from build123d import *

# Parameters (mm, degrees)
SKETCH1_W           = 45
SKETCH1_H           = 70
BOSS_EXTRUDE1_DEPTH = 3
SKETCH2_R           = 10.95
SKETCH2_W           = 24
SKETCH2_H           = 35
CUT_EXTRUDE1_DEPTH  = 4
SKETCH4_W           = 10
SKETCH4_H           = 3
BOSS_EXTRUDE3_DEPTH = 3
SKETCH3_W           = 3
SKETCH3_H           = 14
BOSS_EXTRUDE2_DEPTH = 3
SKETCH5_W           = 45
SKETCH5_H           = 55
BOSS_EXTRUDE4_DEPTH = 3
FILLET1_R           = 4
SKETCH6_R           = 15.5
CUT_EXTRUDE2_DEPTH  = 10


with BuildPart() as part:
    # Sketch1 → Boss-Extrude1 (new body)
    with BuildSketch(Plane.XY):
        Rectangle(SKETCH1_W, SKETCH1_H)
    extrude(amount=BOSS_EXTRUDE1_DEPTH)

    # Sketch2 → Cut-Extrude1 (cut, through all)
    with BuildSketch(Plane.XY.offset(3)):
        with Locations((0, 16)):
            Circle(SKETCH2_R)
        with Locations((0, -17.5)):
            Rectangle(SKETCH2_W, SKETCH2_H)
    extrude(amount=-CUT_EXTRUDE1_DEPTH, mode=Mode.SUBTRACT)

    # Sketch4 → Boss-Extrude3 (add)
    with BuildSketch(Plane.XY.offset(3)):
        with Locations((-10, 36.5)):
            Rectangle(SKETCH4_W, SKETCH4_H)
        with Locations((10, 36.5)):
            Rectangle(SKETCH4_W, SKETCH4_H)
    extrude(amount=-BOSS_EXTRUDE3_DEPTH)

    # Sketch3 → Boss-Extrude2 (add)
    with BuildSketch(Plane(origin=(0, 0, 0), x_dir=(-1, 0, 0), z_dir=(0, 0, -1))):
        with Locations((24, 0)):
            Rectangle(SKETCH3_W, SKETCH3_H)
        with Locations((24, 28)):
            Rectangle(SKETCH3_W, SKETCH3_H)
        with Locations((24, -28)):
            Rectangle(SKETCH3_W, SKETCH3_H)
        with Locations((-24, 14)):
            Rectangle(SKETCH3_W, SKETCH3_H)
        with Locations((-24, -14)):
            Rectangle(SKETCH3_W, SKETCH3_H)
    extrude(amount=-BOSS_EXTRUDE2_DEPTH)

    # Sketch5 → Boss-Extrude4 (add)
    with BuildSketch(Plane.XY.offset(3)):
        with Locations((0, -62.5)):
            Rectangle(SKETCH5_W, SKETCH5_H)
    extrude(amount=-BOSS_EXTRUDE4_DEPTH)

    # Fillet1
    fillet1_edges = [part.edges().sort_by_distance(p)[0] for p in [
        (12, 0, 1.5),
        (12, -35, 1.5),
        (-12, -35, 1.5),
        (-12, 0, 1.5),
    ]]
    fillet(fillet1_edges, radius=FILLET1_R)

    # Sketch6 → Cut-Extrude2 (cut)
    with BuildSketch(Plane(origin=(0, 0, 0), x_dir=(-1, 0, 0), z_dir=(0, 0, -1))):
        with Locations((0, -62.5)):
            Circle(SKETCH6_R)
        with BuildLine():
            Line((13.5, -78), (13.5, -73))
            ThreePointArc((13.5, -73), (15.5, -71), (17.5, -73))
            Line((17.5, -73), (17.5, -78))
            ThreePointArc((17.5, -78), (15.5, -80), (13.5, -78))
        make_face()
        with BuildLine():
            Line((-17.5, -78), (-17.5, -73))
            ThreePointArc((-17.5, -73), (-15.5, -71), (-13.5, -73))
            Line((-13.5, -73), (-13.5, -78))
            ThreePointArc((-13.5, -78), (-15.5, -80), (-17.5, -78))
        make_face()
        with BuildLine():
            Line((-17.5, -47), (-17.5, -42))
            ThreePointArc((-17.5, -42), (-15.5, -40), (-13.5, -42))
            Line((-13.5, -42), (-13.5, -47))
            ThreePointArc((-13.5, -47), (-15.5, -49), (-17.5, -47))
        make_face()
        with BuildLine():
            Line((13.5, -47), (13.5, -42))
            ThreePointArc((13.5, -42), (15.5, -40), (17.5, -42))
            Line((17.5, -42), (17.5, -47))
            ThreePointArc((17.5, -47), (15.5, -49), (13.5, -47))
        make_face()
    extrude(amount=-CUT_EXTRUDE2_DEPTH, mode=Mode.SUBTRACT)


solid = part.part
The model under review builds one solid part; all positions refer to its coordinate system, in mm. A direction names the side the tool comes from. Give positions to 0.01 mm unless a question says otherwise; leave off trailing zeros. Write each loop counter-clockwise with the first axis right and the second up, starting at its lowest first coordinate (ties: lowest second). Pieces come first, ordered by that corner, then holes. Notation, with made-up numbers: M -8.5,-19.75 L 28.5,-19.75 A28 cw 28.5,-0.75 Z; hole C 19.25,23.25 d3. An arc over 180 degrees is marked long. One line per question, with ' | ' between items. Start each with the question number.
Item 1: We need section C-C on x = -20. Write out the cut boundary in (y, z), plus the area to 3 significant figures.
Item 2: Draft analysis for pull direction X (two halves, no side actions). For faces 1 (the flat face through (-5, 36, 2)), 2 (the flat face through (-20, 35, 1)), 3 (the flat face through (-22.5, 14, 1)), 4 (the flat face through (0, 0, 2)), state which applies: released by +X, released by -X, zero draft, split by the parting line, or undercut.
Item 3: For pin 1 (0.9 mm diameter, centred on x = 24.5, z = 1, fed in from -Y); pin 2 (0.9 mm diameter, centred on x = -24.5, z = 1.5, fed in from +Y); pin 3 (6 mm diameter, centred on x = 9.5, y = -16, fed in from -Z); pin 4 (1.5 mm diameter, centred on y = -75.5, z = 2, fed in from -X), all flat-tipped, find the tip position at first contact; note any pin that passes through.
Item 4: We need section B-B on y = 16. Write out the cut boundary in (x, z), plus the area to 3 significant figures.
Item 5: Wall thickness on line 1 (Y direction, x = 0, z = 1.3); line 2 (X direction, y = -42, z = 0.45); line 3 (X direction, y = -8.5, z = 0.25): over which ranges is each line inside the solid? List them lowest first. Write a range as from..to.
Item 6: We need section A-A on y = -44.5. Write out the cut boundary in (x, z).
Item 7: For faces 5 (the flat face through (25.5, 14, 1)), 6 (the flat face through (24, -7, 1)), 7 (the flat face through (0, -35, 2)), 8 (the flat face through (24, -21, 1)), 9 (the flat face through (19, 35, 1)), list the 3-axis set-ups (+Z, -Z, +X, -X, +Y, -Y) from which the entire face can be reached by the end or side of a thin tool; tool diameter is ignored.
Item 8: We need section D-D on z = 1.5. Give the number of separate pieces and of enclosed holes in the cut face, plus the area to 3 significant figures.
Results found:
1) outline: M -90,0 L 35,0 L 35,3 L -90,3 Z | area: 375 mm2
2) face 1: undercut | face 2: zero draft | face 3: released by -X | face 4: undercut
3) pin 1: stops at y = -21 | pin 2: stops at y = 35 | pin 3: stops at z = 0 | pin 4: stops at x = -22.5
4) outline: M -22.5,0 L -10.95,0 L -10.95,3 L -22.5,3 Z; M 10.95,0 L 25.5,0 L 25.5,3 L 10.95,3 Z | area: 78.3 mm2
5) line 1: y = -90..-78, -47..-35, 0..5.05, 26.95..35 | line 2: x = -22.5..-17.5, -13.5..13.5, 17.5..22.5 | line 3: x = -22.5..-12, 12..25.5
6) outline: M -22.5,0 L -17.5,0 L -17.5,3 L -22.5,3 Z; M -13.5,0 L 13.5,0 L 13.5,3 L -13.5,3 Z; M 17.5,0 L 22.5,0 L 22.5,3 L 17.5,3 Z
7) face 5: +Z, -Z, +X, +Y, -Y | face 6: +Z, -Z, +X | face 7: +Z, -Z | face 8: +Z, -Z, +X, -Y | face 9: +Z, -Z, +X, +Y
8) separate pieces: 1 | enclosed holes: 7 | area: 3,810 mm2
